For this review, take the finished solid that the model builds, in its own axes (mm). Face numbers are marked on the shaded views. A direction names the side the tool comes from. Coordinates: 2 decimals unless noted, no trailing zeros. Loops run counter-clockwise (first coordinate to the right, second up) from the corner with the lowest first, then second, coordinate; pieces in that order, holes last. Notation, with made-up numbers: (57.25, 38) -> (67.25, 38) arc R17 ccw to (67.25, 64) -> close; hole circle Ø7 at (14, 45). An arc over 180 degrees is marked (long way). Use a Markdown table: item, result.
from build123d import *

# Parameters (mm, degrees)
SKETCH1_R           = 20
BOSS_EXTRUDE1_DEPTH = 15
SKETCH2_R           = 12.5
BOSS_EXTRUDE2_DEPTH = 23
SKETCH3_R           = 3
CUT_EXTRUDE1_DEPTH  = 48.370877129
FILLET1_R           = 3
CHAMFER1_SIZE       = 0.5
CUT_EXTRUDE2_DEPTH  = 3


with BuildPart() as part:
    # Sketch1 → Boss-Extrude1 (new body)
    with BuildSketch(Plane.XY):
        Circle(SKETCH1_R)
    extrude(amount=BOSS_EXTRUDE1_DEPTH)

    # Sketch2 → Boss-Extrude2 (add)
    with BuildSketch(Plane.XY.offset(15)):
        with Locations((7.5, 0)):
            Circle(SKETCH2_R)
    extrude(amount=BOSS_EXTRUDE2_DEPTH)

    # Sketch3 → Cut-Extrude1 (cut, through all)
    with BuildSketch(Plane.XY.offset(38)):
        with Locations((4, 0)):
            Circle(SKETCH3_R)
    extrude(amount=-CUT_EXTRUDE1_DEPTH, mode=Mode.SUBTRACT)

    # Fillet1
    fillet1_edges = [part.edges().sort_by_distance(p)[0] for p in [
        (-20, 0, 0),
    ]]
    fillet(fillet1_edges, radius=FILLET1_R)

    # Chamfer1
    # the kernel refuses this chamfer: 0.5 mm, written as the material it takes off along each edge
    with BuildSketch(Plane(origin=(0, 0, 15), x_dir=(1, 0, 0), z_dir=(0, -1, 0))) as chamfer1_piece_1_section:
        Polygon((20, -CHAMFER1_SIZE), (20 - CHAMFER1_SIZE, 0), (20, 0), align=None)
    chamfer1_piece_1 = revolve(axis=Axis((0, 0, 15), (0, 0, 1)), mode=Mode.PRIVATE)
    chamfer1_piece_1 = chamfer1_piece_1 - Plane(origin=(7.5, 0, 14.767938502), x_dir=(1, 0, 0), z_dir=(0, 0, -1)) * Cylinder(12.5, 80, mode=Mode.PRIVATE)
    add(chamfer1_piece_1, mode=Mode.SUBTRACT)

    # Sketch5 → Cut-Extrude2 (cut)
    with BuildSketch(Plane.XY.offset(38)):
        with BuildLine():
            Line((7.5, 12.5), (7.5, -12.5))
            ThreePointArc((7.5, -12.5), (-8.980754986, 0), (7.5, 12.5))
        make_face()
    extrude(amount=-CUT_EXTRUDE2_DEPTH, mode=Mode.SUBTRACT)


solid = part.part
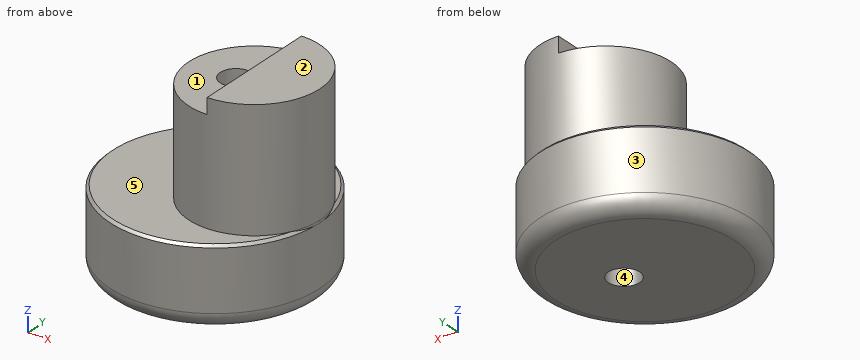
(1) Take a section at A-A on x = 0. Write out the cut boundary in (y, z), plus the area to 3 significant figures.
Found:
| item | result |
|---|---|
| outline | (-20, 3) arc R3 ccw to (-17, 0) -> (17, 0) arc R3 ccw to (20, 3) -> (20, 14.5) -> (19.5, 15) -> (10, 15) -> (10, 35) -> (-10, 35) -> (-10, 15) -> (-19.5, 15) -> (-20, 14.5) -> close |
| area | 996 mm^2 |
(2) For the marked faces 1 and 2, list the 3-axis set-ups (+Z, -Z, +X, -X, +Y, -Y) from which the entire face can be reached by the end or side of a thin tool; tool diameter is ignored.
Found:
| item | result |
|---|---|
| face 1 | +Z, -X, +Y, -Y |
| face 2 | +Z, +X, -X, +Y, -Y |
(3) Take a section at B-B on z = 33. Write out the cut boundary in (x, y), plus the area to 3 significant figures.
Found:
| item | result |
|---|---|
| outline | circle Ø25 at (7.5, 0); hole circle Ø6 at (4, 0) |
| area | 463 mm^2 |
(4) Mouldability with a two-part tool opening along X and no side actions: class the marked faces 3, 4 and 5 as pulls with the +X half, pulls with the -X half, needs draft (parallel to the pull), parting line crosses it, or undercut.
Found:
| item | result |
|---|---|
| face 3 | parting line crosses it |
| face 4 | undercut |
| face 5 | needs draft |
(5) For pin 1 Ø10 at (x, z) = (3.5, 8.5) entering from +Y; pin 2 Ø8 at (y, z) = (9, 5.5) entering from +X; pin 3 Ø1 at (x, y) = (-11.5, -5.5) entering from +Z; pin 4 Ø12 at (y, z) = (-4.5, 4.5) entering from +X, all flat-tipped, find the tip position at first contact; note any pin that passes through.
Found:
| item | result |
|---|---|
| pin 1 | stops at y = 20 |
| pin 2 | stops at x = 19.36 |
| pin 3 | stops at z = 15 |
| pin 4 | stops at x = 20 |
(6) For line 1 along Z through (x, y) = (-6.5, -7); line 2 along Y through (x, z) = (6, 17); line 3 along Y through (x, z) = (3, 4), list the stretches that pass through material, from the lowest coordinate up.
Found:
| item | result |
|---|---|
| line 1 | z = 0 to 15 |
| line 2 | y = -12.41 to -2.24, 2.24 to 12.41 |
| line 3 | y = -19.77 to -2.83, 2.83 to 19.77 |
